Could you check a few things on this model? Use its own coordinates, in mm. A direction names the side the tool comes from. Give positions to 0.01 mm unless a question says otherwise; leave off trailing zeros. Order: outer loops, then holes, each group sorted by start corner. A loop starts at its lowest first (then second) coordinate and runs counter-clockwise, first axis right, second up.
(1) If I drill on probe 1 along X at (y, z) = (20, 8.25); probe 2 along Y at (x, z) = (29.5, 7.75); probe 3 along Y at (x, z) = (-42, 5.5), over which ranges is the centre line in solid material (lowest first)?
(2) On a 3-axis mill with a long thin cutter (end or side, diameter ignored), from which of +Z, -Z, +X, -X, +Y, -Y can I reach the whole of each face in a straight line? I mean faces 5 (the cylindrical face through (45.524, -7.573, 0.301)), 6 (the flat face through (44.3, -7.2, 5.3)). Say none if no direction works.
(3) If we mould it in two halves opening along Y, with no side actions, what happens to faces 1 (the cylindrical face through (-59.64, -22.1, 5.2)), 2 (the flat face through (1, 25, 5)), 3 (the flat face through (-16, -23, 5)), 4 (the flat face through (45.3, -8.2, 4.9))? For each: released by +Y, released by -Y, zero draft, split by the parting line, or undercut.
(4) Imagine slicing it at A-A, the plane z = 7. Write out the boundary of the cut face in (x, y), then the cut area to 3 significant figures.
(5) Imagine slicing it at C-C, the plane x = -2. Write out the boundary of the cut face in (y, z), then the cut area to 3 significant figures.
(6) Imagine slicing it at B-B, the plane y = 15.5. Write out the boundary of the cut face in (x, z).
(7) Will this pin go through, and if not, where does the flat tip stop? pin 1 (1 mm diameter, centred on x = 13, y = 19.5, fed in from +Z).
from build123d import *

# Parameters (mm, degrees)
F1_DEPTH = 9
F3_DEPTH = 8.5
F4_R     = 3
F5_R     = 1


# Not quite as in the source:
# - a feature names something its author has since deleted; it is built from what else it names


with BuildPart() as f1:
    # F0 (on Top) → F1 (new body)
    with BuildSketch(Plane.XY):
        Polygon((-62.5, -25), (28.5, -25), (62.5, 9), (62.5, 25), (-62.5, 25), align=None)
    extrude(amount=F1_DEPTH)

    # F2 (on face) → F3 (cut)
    with BuildSketch(Plane.XY.offset(9)):
        Polygon((60.5, 9), (60.5, 23), (-60.5, 23), (-60.5, -23), (28.5, -23), align=None)
    extrude(amount=-F3_DEPTH, mode=Mode.SUBTRACT)

    # F4
    f4_edges = [f1.edges().sort_by_distance(p)[0] for p in [
        (-60.5, 23, 4.75),
        (60.5, 23, 4.75),
        (60.5, 9, 4.75),
        (28.5, -23, 4.75),
        (-60.5, -23, 4.75),
        (62.5, 25, 4.5),
        (62.5, 9, 4.5),
        (28.5, -25, 4.5),
        (-62.5, 25, 4.5),
        (-62.5, -25, 4.5),
    ]]
    fillet(f4_edges, radius=F4_R)

    # F5
    f5_edges = [f1.edges().sort_by_distance(p)[0] for p in [
        (60.5, 15.12132, 0.5),
        (60.271639, 9.09459, 0.5),
        (59.62132, 22.12132, 0.5),
        (44.5, -7, 0.5),
        (0, 23, 0.5),
        (28.40541, -22.771639, 0.5),
        (-59.62132, 22.12132, 0.5),
        (-15.12132, -23, 0.5),
        (-60.5, 0, 0.5),
        (-59.62132, -22.12132, 0.5),
        (-16.12132, -25, 0),
        (-61.62132, -24.12132, 0),
        (28.40541, -24.771639, 0),
        (-62.5, 0, 0),
        (45.5, -8, 0),
        (-61.62132, 24.12132, 0),
        (62.271639, 9.09459, 0),
        (0, 25, 0),
        (62.5, 16.12132, 0),
        (61.62132, 24.12132, 0),
    ]]
    fillet(f5_edges, radius=F5_R)


solid = f1.part
Answer block:
1. probe 1: x = -62.5 to -60.5, 60.5 to 62.5
1. probe 2: y = -24 to -22, 23 to 25
1. probe 3: y = -25 to -23, 23 to 25
2. face 5: -Z, +X, -Y
2. face 6: +Z
3. face 1: undercut
3. face 2: released by +Y
3. face 3: undercut
3. face 4: released by -Y
4. outline: (-62.5, -22) arc R3 ccw to (-59.5, -25) - (27.26, -25) arc R3 ccw to (29.38, -24.12) - (61.62, 8.12) arc R3 ccw to (62.5, 10.24) - (62.5, 22) arc R3 ccw to (59.5, 25) - (-59.5, 25) arc R3 ccw to (-62.5, 22) - close; hole (-60.5, -20) arc R3 ccw to (-57.5, -23) - (27.26, -23) arc R3 ccw to (29.38, -22.12) - (59.62, 8.12) arc R3 ccw to (60.5, 10.24) - (60.5, 20) arc R3 ccw to (57.5, 23) - (-57.5, 23) arc R3 ccw to (-60.5, 20) - close
4. area: 618 mm2
5. outline: (-25, 1) arc R1 ccw to (-24, 0) - (24, 0) arc R1 ccw to (25, 1) - (25, 9) - (23, 9) - (23, 1.5) arc R1 cw to (22, 0.5) - (-22, 0.5) arc R1 cw to (-23, 1.5) - (-23, 9) - (-25, 9) - close
5. area: 59.0 mm2
6. outline: (-62.5, 1) arc R1 ccw to (-61.5, 0) - (61.5, 0) arc R1 ccw to (62.5, 1) - (62.5, 9) - (60.5, 9) - (60.5, 1.5) arc R1 cw to (59.5, 0.5) - (-59.5, 0.5) arc R1 cw to (-60.5, 1.5) - (-60.5, 9) - (-62.5, 9) - close
7. pin 1: stops at z = 0.5
